Autodesk Inventor part; units mm, degrees
ref_plane "YZ Plane" through (0, 0, 0) normal (1, 0, 0) x (0, 1, 0)
ref_plane "XZ Plane" through (0, 0, 0) normal (0, 1, 0) x (-1, 0, 0)
ref_plane "XY Plane" through (0, 0, 0) normal (0, 0, 1) x (1, 0, 0)
sketch "Sketch1" plane through (0, 0, 0) normal (0, 1, 0) x (-1, 0, 0)
  circle A0 centre (0, 0) radius 1.5875
  circle A1 centre (0, 0) radius 6.35
  dimension "d0" = 3.175
  dimension "d1" = 12.7
extrude "Extrusion1" add sketch "Sketch1" along normal blind 5.08 contours A0 | A1
extrude "Extrusion2" add sketch "Sketch1" against normal blind 12.7 contours A0
sketch "Sketch2" plane through (0, 5.08, 0) normal (0, 1, 0) x (1, 0, 0)
  line L0 (6.3393, 0) -> (3.5604, 1.4472)
  line L1 (3.5604, 1.4472) -> (6.3393, 0)
  line L2 (6.3393, 0) -> (3.381, -1.08)
  line L3 (0, 0) -> (-1.7844, 0)
  circle A0 centre (0, 0) radius 6.35
  line L4 (0, -6.35) -> (1.3494, -3.7028)
  line L5 (0, -6.35) -> (-0.8922, -3.6818)
  line L6 (-6.35, 0) -> (-3.4749, -1.7844)
  line L7 (-3.4749, -1.7844) -> (-6.35, 0)
  line L8 (-3.6501, 1.1418) -> (-6.35, 0)
  line L9 (0, 6.35) -> (1.509, 4.0476)
  line L10 (1.509, 4.0476) -> (0, 6.35)
  line L11 (0, 6.35) -> (-1.2759, 3.8681)
  line L12 (1.509, 4.0476) -> (4.4233, 4.556)
  line L13 (3.5604, 1.4472) -> (4.4233, 4.556)
  line L14 (3.381, -1.08) -> (4.4233, -4.556)
  line L15 (1.3494, -3.7028) -> (4.4233, -4.556)
  line L16 (-0.8922, -3.6818) -> (-3.4749, -5.0301)
  line L17 (-3.4749, -5.0301) -> (-3.4749, -1.7844)
  line L18 (-3.6501, 1.1418) -> (-4.2707, 4.6993)
  line L19 (-1.2759, 3.8681) -> (-4.2707, 4.6993)
  circle A1 centre (0, 0) radius 6.35
extrude "Extrusion3" cut sketch "Sketch2" against normal blind 5.08 contours L0 L13 A0 L14 L2 | L12 L9 A0 | A0 L4 L15 | L11 L19 A0 | A0 L6 L17 L16 L5 | L18 L8 A0
properties part number "Wheels" material "PBT Plastic"
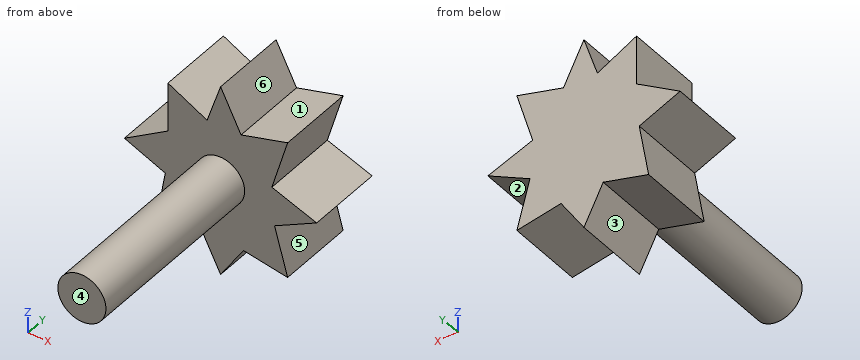
Check sheet for the modelled part. Datum: model origin and axes. Units: mm. Face numbers are marked on the shaded views. A direction names the side the tool comes from. Round coordinates to 2 decimals unless told otherwise and drop trailing zeros. Loops run counter-clockwise (first coordinate to the right, second up) from the corner with the lowest first, then second, coordinate; pieces in that order, holes last. Notation, with made-up numbers: (-29.75, -13.5) -> (23.25, -13.5) arc R18 cw to (23.25, -2.5) -> close; hole circle Ø2 at (84, 48.25). An arc over 180 degrees is marked (long way). Put each result on its own line as item: value. Start each with the question number.
1. Section check D-D (z = 2.75). Enter the section's corners in (x, y), plus the area to 3 significant figures.
2. Gauge pin test, flat ends, axial feed: pin 1 (3.5 mm diameter, centred on y = 2, z = 3.5, fed in from -X); pin 2 (5 mm diameter, centred on x = 2.5, y = -7, fed in from -Z); pin 3 (4 mm diameter, centred on y = -0.5, z = -5, fed in from +X). Record the tip position at first contact, or that the pin passes through.
3. Section check A-A (x = 4). Enter the section's corners in (y, z).
4. Section check B-B (y = 4). Enter the section's corners in (x, z).
5. Section check C-C (x = -4.75). Enter the section's corners in (y, z), plus the area to 3 significant figures.
6. Access from +Z, -Z, +X, -X, +Y, -Y to the whole of each face (thin tool, end or side, straight path). Record for the marked faces 1, 2 and 3.
7. Draft check along Z on the marked faces 4, 5 and 6. Enter one of: +Z half, -Z half, draft (parallel to the pull), parting line (faces both ways), or undercut.
8. Scan lines: probe 1 along Y at (x, z) = (3.75, 0.5); probe 2 along Z at (x, y) = (5.75, 1.25); probe 3 along X at (y, z) = (4, 3.25). Record each from-to range of solid material in increasing order.
Findings:
1. outline: (-3.47, 0) -> (3.88, 0) -> (3.88, 5.08) -> (-3.47, 5.08) -> close
1. area: 37.4 mm^2
2. pin 1: stops at x = -3.53
2. pin 2: stops at z = -1.59
2. pin 3: stops at x = 4.42
3. outline: (0, -4.48) -> (5.08, -4.48) -> (5.08, -3.03) -> (0, -3.03) -> close; (0, -1.22) -> (5.08, -1.22) -> (5.08, 0.85) -> (0, 0.85) -> close; (0, 3.14) -> (5.08, 3.14) -> (5.08, 4.44) -> (0, 4.44) -> close
4. outline: (-6.35, 0) -> (-3.65, -1.14) -> (-4.27, -4.7) -> (-1.28, -3.87) -> (0, -6.35) -> (1.51, -4.05) -> (4.42, -4.56) -> (3.56, -1.45) -> (6.34, 0) -> (3.38, 1.08) -> (4.42, 4.56) -> (1.35, 3.7) -> (0, 6.35) -> (-0.89, 3.68) -> (-3.47, 5.03) -> (-3.47, 1.78) -> close
5. outline: (0, -0.68) -> (5.08, -0.68) -> (5.08, 0.99) -> (0, 0.99) -> close
5. area: 8.48 mm^2
6. face 1: +Z, +Y, -Y
6. face 2: +X, +Y, -Y
6. face 3: -Z, +Y, -Y
7. face 4: draft
7. face 5: undercut
7. face 6: +Z half
8. probe 1: y = 0 to 5.08
8. probe 2: z = -0.31 to 0.22
8. probe 3: x = -3.47 to 4.03
